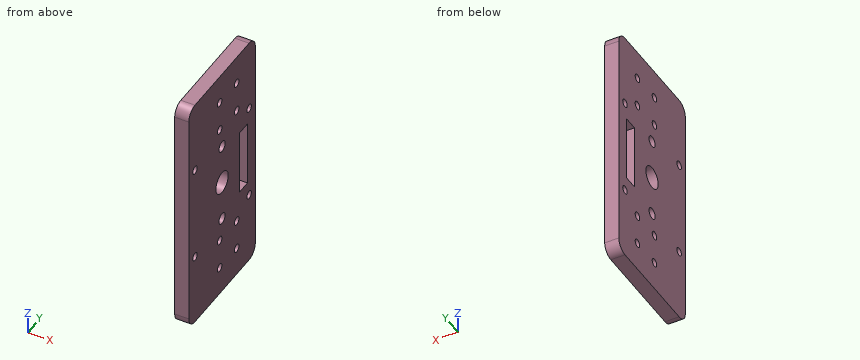
```python
from build123d import *

# Parameters (mm, degrees)
SKETCH1_W              = 110
SKETCH1_H              = 54
BOSS_EXTRUDE1_DEPTH    = 6.35
FILLET1_R              = 5
F_6_CLEARANCE_HOLE1_D  = 3.6576
SKETCH5_R              = 5
CUT_EXTRUDE1_DEPTH     = 7.35
F_6_CLEARANCE_HOLE2_D  = 3.6576
SKETCH10_W             = 30
SKETCH10_H             = 6.35
CUT_EXTRUDE2_DEPTH     = 7.35
F_10_CLEARANCE_HOLE1_D = 4.9784


with BuildPart() as part:
    # Sketch1 → Boss-Extrude1 (new body)
    with BuildSketch(Plane(origin=(0, 0, 0), x_dir=(0, 0, -1), z_dir=(1, 0, 0))):
        Rectangle(SKETCH1_W, SKETCH1_H)
    extrude(amount=BOSS_EXTRUDE1_DEPTH)

    # Fillet1
    fillet1_edges = [part.edges().sort_by_distance(p)[0] for p in [
        (3.175, -27, -55),
        (3.175, -27, 55),
        (3.175, 27, 55),
        (3.175, 27, -55),
    ]]
    fillet(fillet1_edges, radius=FILLET1_R)

    # #6 Clearance Hole1 (through all)
    with Locations(Plane(origin=(6.35, 0, 0), x_dir=(0, 0, -1), z_dir=(1, 0, 0))):
        with Locations((-22, 22), (22, 22), (22, -22), (-22, -22)):
            Hole(F_6_CLEARANCE_HOLE1_D / 2)

    # Sketch5 → Cut-Extrude1 (cut, through all)
    with BuildSketch(Plane(origin=(6.35, 0, 0), x_dir=(0, 0, -1), z_dir=(1, 0, 0))):
        Circle(SKETCH5_R)
    extrude(amount=-CUT_EXTRUDE1_DEPTH, mode=Mode.SUBTRACT)

    # #6 Clearance Hole2 (through all)
    with Locations(Plane(origin=(6.35, 0, 0), x_dir=(0, 0, -1), z_dir=(1, 0, 0))):
        with Locations((-41.914797213, 11.884797213), (-28.085202787, 11.884797213), (-28.085202787, -1.944797213), (-41.914797213, -1.944797213), (28.085202787, 11.884797213), (28.085202787, -1.944797213), (41.914797213, -1.944797213), (41.914797213, 11.884797213)):
            Hole(F_6_CLEARANCE_HOLE2_D / 2)

    # Sketch10 → Cut-Extrude2 (cut, through all)
    with BuildSketch(Plane.ZY):
        with Locations((0, 17.475)):
            Rectangle(SKETCH10_W, SKETCH10_H)
    extrude(amount=-CUT_EXTRUDE2_DEPTH, mode=Mode.SUBTRACT)

    # #10 Clearance Hole1 (through all)
    with Locations(Plane.ZY):
        with Locations((18.25, 0), (-18.25, 0)):
            Hole(F_10_CLEARANCE_HOLE1_D / 2)


solid = part.part
```
Check sheet for the modelled part. Datum: model origin and axes. Units: mm. Round coordinates to 2 decimals unless told otherwise and drop trailing zeros. Loops run counter-clockwise (first coordinate to the right, second up) from the corner with the lowest first, then second, coordinate; pieces in that order, holes last. Notation, with made-up numbers: (-0.5, 3) -> (32.5, 3) arc R23 cw to (32.5, 11) -> close; hole circle Ø1 at (-40, 82). An arc over 180 degrees is marked (long way). Write item = value, one per line. Start each with the question number.
1) Sectioned sample at C-C, the plane z = 0. Record the cut outline in (x, y).
2) Gauge pin test, flat end, axial feed: pin 1 Ø3.5 at (y, z) = (-1.94, -28.09) entering from -X. Record the tip position at first contact, or that the pin passes through.
3) Thickness scan on probe 1 along Y at (x, z) = (3, 40.5); probe 2 along Z at (x, y) = (3.25, 1.5); probe 3 along Y at (x, z) = (1.5, 29). Record the ranges inside material, lowest first.
4) Sectioned sample at D-D, the plane y = 1.5. Record the cut outline in (x, z).
5) Sectioned sample at B-B, the plane y = 18. Record the cut outline in (x, z).
6) Sectioned sample at A-A, the plane z = 18.25. Record the cut outline in (x, y), plus the area to 3 significant figures.
Results are:
q1.outline = (0, -27) -> (6.35, -27) -> (6.35, -5) -> (0, -5) -> close; (0, 5) -> (6.35, 5) -> (6.35, 14.3) -> (0, 14.3) -> close; (0, 20.65) -> (6.35, 20.65) -> (6.35, 27) -> (0, 27) -> close
q2.pin_1 = through
q3.probe_1 = -27 to -3.1, -0.79 to 10.73, 13.04 to 27
q3.probe_2 = -55 to -20.24, -16.26 to -4.77, 4.77 to 16.26, 20.24 to 55
q3.probe_3 = -27 to -3.53, -0.36 to 10.3, 13.47 to 27
q4.outline = (0, -55) -> (6.35, -55) -> (6.35, -20.24) -> (0, -20.24) -> close; (0, -16.26) -> (6.35, -16.26) -> (6.35, -4.77) -> (0, -4.77) -> close; (0, 4.77) -> (6.35, 4.77) -> (6.35, 16.26) -> (0, 16.26) -> close; (0, 20.24) -> (6.35, 20.24) -> (6.35, 55) -> (0, 55) -> close
q5.outline = (0, -55) -> (6.35, -55) -> (6.35, -15) -> (0, -15) -> close; (0, 15) -> (6.35, 15) -> (6.35, 55) -> (0, 55) -> close
q6.outline = (0, -27) -> (6.35, -27) -> (6.35, -2.49) -> (0, -2.49) -> close; (0, 2.49) -> (6.35, 2.49) -> (6.35, 27) -> (0, 27) -> close
q6.area = 311 mm^2
